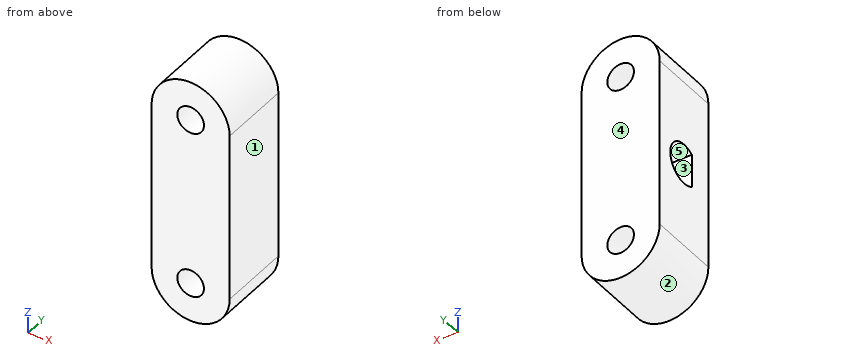
```python
from build123d import *

# Parameters (mm, degrees)
EXTRUDE_1_DEPTH     = 11
SKETCH_2_R          = 2.05
CUT_EXTRUDE_1_DEPTH = 12
SKETCH_3_R          = 3.1
CUT_EXTRUDE_2_DEPTH = 10
EXTRUDE_3_DEPTH     = 10


with BuildPart() as part:
    # 草图1 → 凸台-拉伸1 (new body)
    with BuildSketch(Plane(origin=(0, 0, 0), x_dir=(1, 0, 0), z_dir=(0, 1, 0))):
        with BuildLine():
            Line((-6, -13), (-6, 13))
            ThreePointArc((-6, 13), (0, 19), (6, 13))
            Line((6, 13), (6, -13))
            ThreePointArc((6, -13), (0, -19), (-6, -13))
        make_face()
    extrude(amount=EXTRUDE_1_DEPTH)

    # 草图2 → 切除-拉伸1 (cut, through all)
    with BuildSketch(Plane(origin=(0, 11, 0), x_dir=(1, 0, 0), z_dir=(0, 1, 0))):
        with Locations((0, 13)):
            Circle(SKETCH_2_R)
        with Locations((0, -13)):
            Circle(SKETCH_2_R)
    extrude(amount=-CUT_EXTRUDE_1_DEPTH, mode=Mode.SUBTRACT)

    # 草图3 → 切除-拉伸2 (cut)
    with BuildSketch(Plane.ZY.offset(6)):
        with Locations((0, 5.5)):
            Circle(SKETCH_3_R)
    extrude(amount=-CUT_EXTRUDE_2_DEPTH, mode=Mode.SUBTRACT)

    # 草图4 → 凸台-拉伸3 (add)
    with BuildSketch(Plane.ZY.offset(6)):
        with BuildLine():
            Line((3.146029243, 3.75), (-3.146029243, 3.75))
            ThreePointArc((-3.146029243, 3.75), (0, 1.9), (3.146029243, 3.75))
        make_face()
    extrude(amount=-EXTRUDE_3_DEPTH)


solid = part.part
```
Geometry: final body of the model. Coordinates: model frame, mm. Face numbers are marked on the shaded views. A direction names the side the tool comes from. Round coordinates to 2 decimals unless told otherwise and drop trailing zeros. Order: outer loops, then holes, each group sorted by start corner. A loop starts at its lowest first (then second) coordinate and runs counter-clockwise, first axis right, second up. Notation, with made-up numbers: M -34,65 L -20,65 A33 cw -20,103 Z; hole C 21.5,-15 d5. An arc over 180 degrees is marked long. Use one line per item in the form item = value. Start each with the question number.
Q1. Cut plane A-A (x = 0). Return loops of the section in (y, z), and give its area (3 significant figures).
Q2. Access query for the marked faces 4 and 5. Directions: +Z, -Z, +X, -X, +Y, -Y. A direction counts if a zero-diameter tool reaches every point of the face in a straight line with its end or side. Return the directions, or none.
Q3. Cut plane D-D (x = -5). Return loops of the section in (y, z), and give its area (3 significant figures).
Q4. Cut plane B-B (y = 7.25). Return loops of the section in (x, z), and give its area (3 significant figures).
Q5. Cut plane C-C (z = 0). Return loops of the section in (x, y).
Q6. Material intervals for line 1 (Z direction, x = 0, y = 0.75); line 2 (X direction, y = 4.25, z = -13); line 3 (Z direction, x = 0.75, y = 2.75), sorted ascending. Write a range as [from, to].
Q7. Mould query, pull axis Z, two halves, no side actions, for the marked faces 1, 2 and 3. Classes: +Z half, -Z half, draft (parallel to the pull), parting line (faces both ways), or undercut.
Q8. Pin query (flat end, axial travel): pin 1 Ø2.5 at (x, z) = (0, 13) entering from +Y. Return the tip coordinate at first contact, or that it passes through.
Geometry results:
q1.outline = M 0,-19 L 11,-19 L 11,-15.05 L 0,-15.05 Z; M 0,-10.95 L 11,-10.95 L 11,10.95 L 0,10.95 Z; M 0,15.05 L 11,15.05 L 11,19 L 0,19 Z; hole M 3.75,-2.56 A3.1 ccw long 3.75,2.56 Z
q1.area = 302 mm^2
q2.face_4 = +Z, -Z, +X, -X, +Y
q2.face_5 = -X
q3.outline = M 0,-16.32 L 11,-16.32 L 11,16.32 L 0,16.32 Z; hole M 3.75,-2.56 A3.1 ccw long 3.75,2.56 Z
q3.area = 334 mm^2
q4.outline = M -6,-13 A6 ccw 6,-13 L 6,13 A6 ccw -6,13 L -6,2.56 L 4,2.56 L 4,-2.56 L -6,-2.56 Z; hole C 0,-13 d4.1; hole C 0,13 d4.1
q4.area = 348 mm^2
q5.outline = M -6,0 L 6,0 L 6,11 L -6,11 L -6,8.6 L 4,8.6 L 4,3.75 L -6,3.75 Z
q6.line_1 = [-19, -15.05], [-10.95, 10.95], [15.05, 19]
q6.line_2 = [-6, -2.05], [2.05, 6]
q6.line_3 = [-18.95, -14.91], [-11.09, 11.09], [14.91, 18.95]
q7.face_1 = draft
q7.face_2 = -Z half
q7.face_3 = undercut
q8.pin_1 = through
